from build123d import *

# Parameters (mm, degrees)
F0_R     = 38.1
F0_W     = 50.8
F0_H     = 50.8
F0_R_2   = 12.7
F1_DEPTH = 12.7
F2_W     = 50.8
F2_H     = 50.8
F3_DEPTH = 25.4
F4_R     = 12.7
F5_DEPTH = 25.4


with BuildPart() as f1:
    # F0 (on Top) → F1 (new body)
    with BuildSketch(Plane.XY):
        Circle(F0_R)
        Rectangle(F0_W, F0_H, mode=Mode.SUBTRACT)
        Rectangle(F0_W, F0_H)
        Circle(F0_R_2, mode=Mode.SUBTRACT)
        Circle(F0_R_2)
    extrude(amount=F1_DEPTH)

    # F2 (on Top) → F3 (join)
    with BuildSketch(Plane.XY):
        Rectangle(F2_W, F2_H)
    extrude(amount=F3_DEPTH)

    # F4 (on Top) → F5 (cut)
    with BuildSketch(Plane.XY):
        Circle(F4_R)
    extrude(amount=F5_DEPTH, mode=Mode.SUBTRACT)


solid = f1.part
Design review of the part built by this model. Coordinates are the model's own, in mm. A direction names the side the tool comes from. Coordinates: 2 decimals unless noted, no trailing zeros. Order: outer loops, then holes, each group sorted by start corner. A loop starts at its lowest first (then second) coordinate and runs counter-clockwise, first axis right, second up.
Item 1: For line 1 (Y direction, x = 0, z = 18); line 2 (Y direction, x = 0, z = 7); line 3 (Z direction, x = -16, y = -28.5), list the stretches that pass through material, from the lowest coordinate up.
Item 2: For pin 1 Ø2 at (y, z) = (8, 22) entering from +X; pin 2 Ø8 at (y, z) = (-14.5, 18.5) entering from -X; pin 3 Ø6.5 at (x, z) = (-7, 19.5) entering from -Y, all flat-tipped, find the tip position at first contact; note any pin that passes through.
Item 3: The part is to be moulded in two halves that separate along Y. For faces 1 (the flat face through (0, -25.4, 19)), 2 (the flat face through (16, 1, 0)), 3 (the cylindrical face through (-2.75, -12.4, 12.52)), say which applies: pulls with the +Y half, pulls with the -Y half, needs draft (parallel to the pull), parting line crosses it, or undercut.
Item 4: Take a section at A-A, the plane x = 0. Write out the cut boundary in (y, z).
Item 5: For faces 4 (the flat face through (-25.4, 0, 19)), 5 (the flat face through (0, 25.4, 19)), 6 (the flat face through (25.4, 0, 19)), list the 3-axis set-ups (+Z, -Z, +X, -X, +Y, -Y) from which the entire face can be reached by the end or side of a thin tool; tool diameter is ignored.
Item 6: Take a section at D-D, the plane y = 19. Write out the cut boundary in (x, z).
Item 7: Take a section at C-C, the plane z = 14. Write out the cut boundary in (x, y).
The answers:
1. line 1: y = -25.4 to -12.7, 12.7 to 25.4
1. line 2: y = -38.1 to -12.7, 12.7 to 38.1
1. line 3: z = 0 to 12.7
2. pin 1: stops at x = 25.4
2. pin 2: stops at x = -25.4
2. pin 3: stops at y = -25.4
3. face 1: pulls with the -Y half
3. face 2: needs draft
3. face 3: undercut
4. outline: (-38.1, 0) - (-12.7, 0) - (-12.7, 25.4) - (-25.4, 25.4) - (-25.4, 12.7) - (-38.1, 12.7) - close; (12.7, 0) - (38.1, 0) - (38.1, 12.7) - (25.4, 12.7) - (25.4, 25.4) - (12.7, 25.4) - close
5. face 4: +Z, -X, +Y, -Y
5. face 5: +Z, +X, -X, +Y
5. face 6: +Z, +X, +Y, -Y
6. outline: (-33.02, 0) - (33.02, 0) - (33.02, 12.7) - (25.4, 12.7) - (25.4, 25.4) - (-25.4, 25.4) - (-25.4, 12.7) - (-33.02, 12.7) - close
7. outline: (-25.4, -25.4) - (25.4, -25.4) - (25.4, 25.4) - (-25.4, 25.4) - close; hole circle Ø25.4 at (0, 0)
